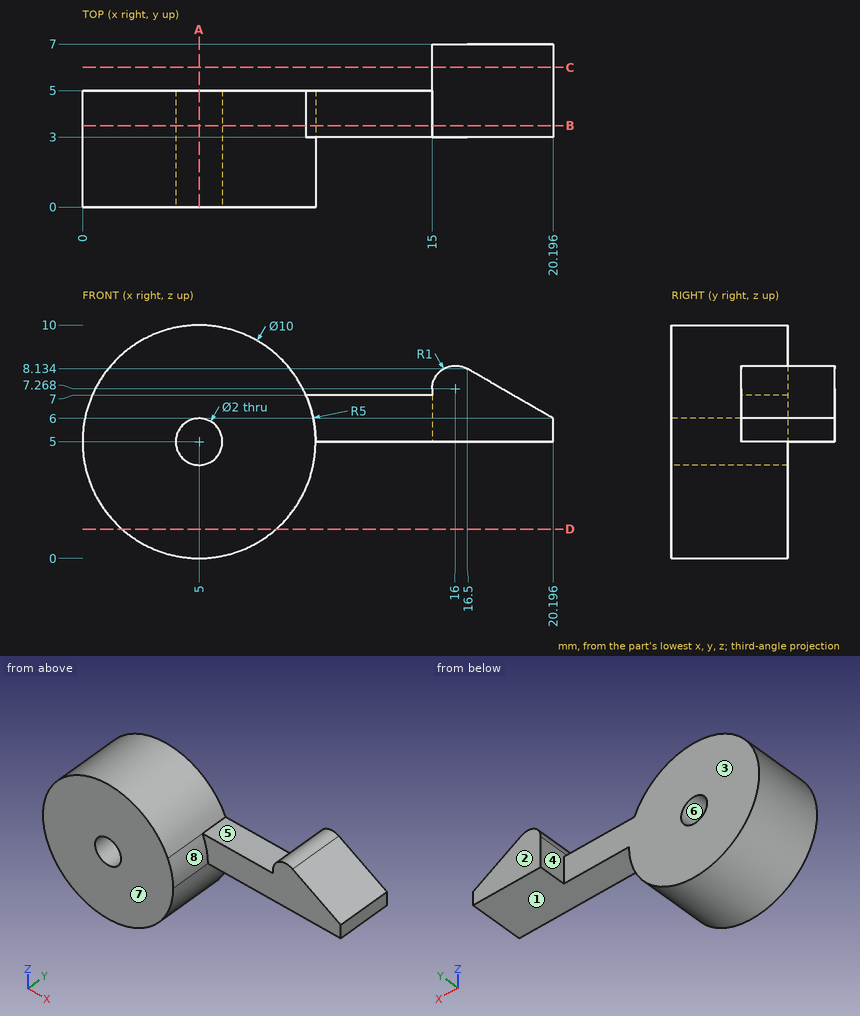
Design review of the part shown in the three views and the two pictorial views. Dimensions are in mm from the part's minimum x, y and z. A direction names the side the tool comes from. Round coordinates to 2 decimals unless told otherwise and drop trailing zeros. Write each loop counter-clockwise with the first axis right and the second up, starting at its lowest first coordinate (ties: lowest second). Pieces come first, ordered by that corner, then holes.
1) Take a section at D-D on z = 1.25. Give the boundary of the cut face in (x, y), then the cut area to 3 significant figures.
Answer below:
outline: (1.69, 0) - (8.31, 0) - (8.31, 5) - (1.69, 5) - close
area: 33.1 mm2
2) Take a section at A-A on x = 5. Give the boundary of the cut face in (y, z).
Answer below:
outline: (0, 0) - (5, 0) - (5, 4) - (0, 4) - close; (0, 6) - (5, 6) - (5, 10) - (0, 10) - close
3) Insertion check: pin 1 Ø1.6 at (x, y) = (12.5, 4.5) entering from +Z; pin 2 Ø6 at (x, z) = (13.5, 6) entering from -Y; pin 3 Ø1.6 at (x, z) = (5, 5) entering from +Y; pin 4 Ø1.2 at (x, y) = (14, 4.5) entering from -Z. Each pin has a flat end and moves straight along its axis. Give the tip position at first contact, or say it passes through.
Answer below:
pin 1: stops at z = 7
pin 2: stops at y = 3
pin 3: passes through
pin 4: stops at z = 5
4) Machinability: for the marked faces 1, 2, 3 and 4, which of the approach directions +Z, -Z, +X, -X, +Y, -Y give a long, thin tool a straight path to every point of the face, cutting with its end or side? Answer none if there is none.
Answer below:
face 1: -Z, +X, +Y, -Y
face 2: +Z, -Z, +X, -X, +Y
face 3: +Z, -Z, -X, +Y
face 4: +Z, +Y
5) Take a section at C-C on y = 6. Give the boundary of the cut face in (x, z), then the cut area to 3 significant figures.
Answer below:
outline: (15, 5) - (20.2, 5) - (20.2, 6) - (16.5, 8.13) arc R1 ccw to (15, 7.27) - close
area: 12.3 mm2
6) For line 1 along Z through (x, y) = (5, 2.35); line 2 along Z through (x, y) = (16, 6.25); line 3 along Y through (x, z) = (8.5, 7.5), list the stretches that pass through material, from the lowest coordinate up.
Answer below:
line 1: z = 0 to 4, 6 to 10
line 2: z = 5 to 8.27
line 3: y = 0 to 5
7) Mouldability with a two-part tool opening along X and no side actions: class the marked faces 5, 6, 7 and 8 as +X half, -X half, draft (parallel to the pull), parting line (faces both ways), or undercut.
Answer below:
face 5: undercut
face 6: undercut
face 7: draft
face 8: +X half
8) Take a section at B-B on y = 3.5. Give the boundary of the cut face in (x, z).
Answer below:
outline: (9.58, 7) arc R5 ccw (long way) to (10, 5) - (20.2, 5) - (20.2, 6) - (16.5, 8.13) arc R1 ccw to (15, 7.27) - (15, 7) - close; hole circle Ø2 at (5, 5)
